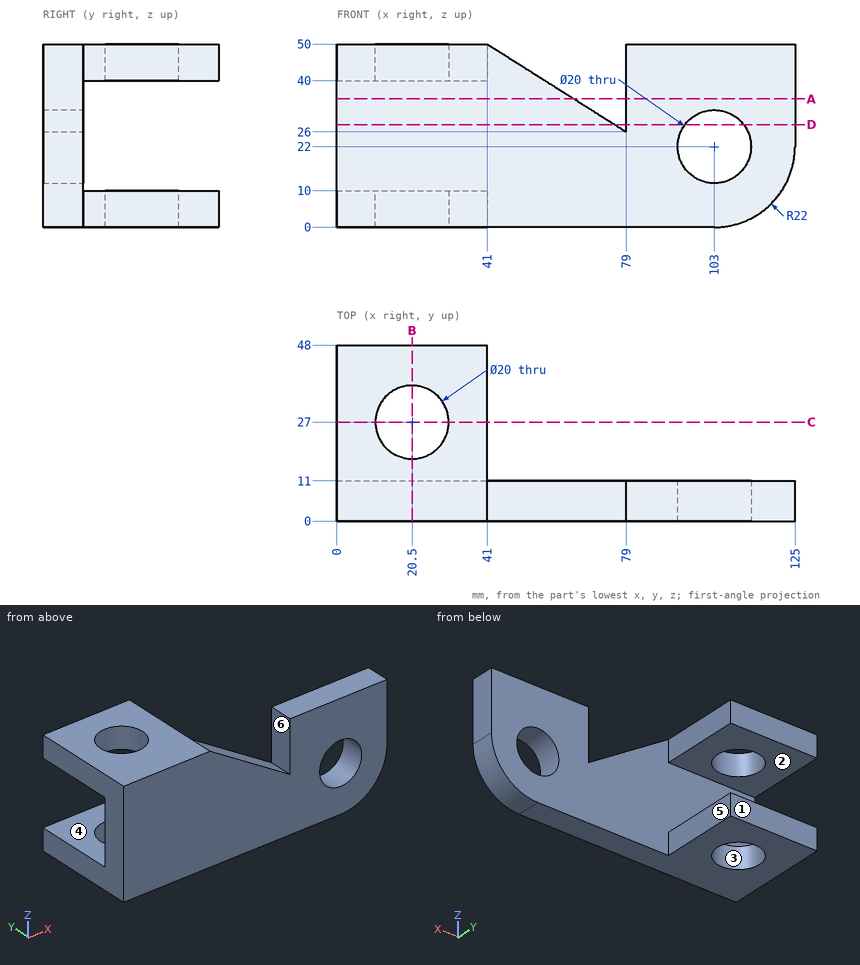
Can you work these out from the drawing? Everything is in mm from the part's minimum corner. A direction names the side the tool comes from. Round coordinates to 2 decimals unless told otherwise and drop trailing zeros. Loops run counter-clockwise (first coordinate to the right, second up) from the corner with the lowest first, then second, coordinate; pieces in that order, holes last. Notation, with made-up numbers: (31, 49) - (85, 49) arc R18 cw to (85, 80) - close; hole circle Ø4 at (28.5, -16). An arc over 180 degrees is marked (long way). Write item = value, one per line. Start each with the question number.
(1) If we section it at A-A (z = 35): Please give me the cut outline in (x, y).
(2) If I drill on probe 1 along Y at (x, z) = (20, 4); probe 2 along Z at (x, y) = (103, 7); probe 3 along Y at (x, z) = (13, 36.5), over which ranges is the centre line in solid material (lowest first)? Write a range as [from, to].
(3) If we section it at B-B (x = 20.5): Please give me the cut outline in (y, z), and give its area (3 significant figures).
(4) If we section it at D-D (z = 28): Please give me the cut outline in (x, y), and give its area (3 significant figures).
(5) For the marked faces 4, 5 and 6, which set-ups out of +Z, -Z, +X, -X, +Y, -Y let a thin tool reach every point of the face, with its end or its side?
(6) For P1, Ø5, axis at y = 24, z = 44, coming from the +X side; P2, Ø25, axis at x = 92.5, z = 26.5, coming from the +Y side, each with a flat end and sliding along its axis, tell me the tip position at first contact or that it passes through.
(7) If we section it at C-C (y = 27): Please give me the cut outline in (x, z), and give its area (3 significant figures).
(8) If we mould it in two halves opening along Y, with no side actions, what happens to the marked faces 1, 2 and 3? For each: released by +Y, released by -Y, zero draft, split by the parting line, or undercut.
Ans:
q1.outline = (0, 0) - (64.75, 0) - (64.75, 11) - (0, 11) - close; (79, 0) - (125, 0) - (125, 11) - (79, 11) - close
q2.probe_1 = [0, 17.01], [36.99, 48]
q2.probe_2 = [0, 12], [32, 50]
q2.probe_3 = [0, 11]
q3.outline = (0, 0) - (17, 0) - (17, 10) - (11, 10) - (11, 40) - (17, 40) - (17, 50) - (0, 50) - close; (37, 0) - (48, 0) - (48, 10) - (37, 10) - close; (37, 40) - (48, 40) - (48, 50) - (37, 50) - close
q3.area = 890 mm²
q4.outline = (0, 0) - (75.83, 0) - (75.83, 11) - (0, 11) - close; (79, 0) - (95, 0) - (95, 11) - (79, 11) - close; (111, 0) - (125, 0) - (125, 11) - (111, 11) - close
q4.area = 1,160 mm²
q5.face_4 = +X, -X, +Y
q5.face_5 = +Z, -Z, +X, +Y
q5.face_6 = +Z, +Y, -Y
q6.P1 = 41
q6.P2 = 11
q7.outline = (0, 0) - (10.5, 0) - (10.5, 10) - (0, 10) - close; (0, 40) - (10.5, 40) - (10.5, 50) - (0, 50) - close; (30.5, 0) - (41, 0) - (41, 10) - (30.5, 10) - close; (30.5, 40) - (41, 40) - (41, 50) - (30.5, 50) - close
q7.area = 420 mm²
q8.face_1 = released by +Y
q8.face_2 = zero draft
q8.face_3 = undercut
